Design review of the part built by this model. Coordinates are the model's own, in mm. Face numbers are marked on the shaded views. A direction names the side the tool comes from. Round coordinates to 2 decimals unless told otherwise and drop trailing zeros. Loops run counter-clockwise (first coordinate to the right, second up) from the corner with the lowest first, then second, coordinate; pieces in that order, holes last. Notation, with made-up numbers: M 23.25,36 L 52.25,36 A19 ccw 52.25,65 Z; hole C 62,58 d7. An arc over 180 degrees is marked long. Use a Markdown table: item, result.
from build123d import *

# Parameters (mm, degrees)
BOSS_EXTRU_1_DEPTH      = 10
ESQUISSE2_R             = 8.5
BOSS_EXTRU_2_DEPTH      = 15
BOSS_EXTRU_2_DEPTH_BACK = 25


with BuildPart() as part:
    # Esquisse1 → Boss.-Extru.1 (new body)
    with BuildSketch(Plane.XY):
        with BuildLine():
            Line((-38.999653337, 10.226454502), (-81.337427048, -4.313992939))
            ThreePointArc((-81.337427048, -4.313992939), (-86.130996021, -4.736088564), (-90.566704705, -2.870356351))
            Line((-90.566704705, -2.870356351), (-108.115218138, 10.226454502))
            ThreePointArc((-108.115218138, 10.226454502), (-118.115218138, 20.226454502), (-108.115218138, 30.226454502))
            Line((-108.115218138, 30.226454502), (61.31386316, 30.226454502))
            ThreePointArc((61.31386316, 30.226454502), (68.788631458, 33.322604906), (71.884781862, 40.797373204))
            Line((71.884781862, 40.797373204), (71.884781862, 45.226454502))
            ThreePointArc((71.884781862, 45.226454502), (81.607354933, 55.230528024), (91.884781862, 45.797373204))
            Line((91.884781862, 45.797373204), (91.884781862, 20.226454502))
            ThreePointArc((91.884781862, 20.226454502), (88.955849674, 13.15538669), (81.884781862, 10.226454502))
            Line((81.884781862, 10.226454502), (-38.999653337, 10.226454502))
        make_face()
    extrude(amount=BOSS_EXTRU_1_DEPTH)

    # Esquisse2 → Boss.-Extru.2 (add, two sides)
    with BuildSketch(Plane.XY.offset(10)) as boss_extru_2_sk:
        with Locations((-108.115218138, 20.226454502)):
            Circle(ESQUISSE2_R)
    extrude(amount=BOSS_EXTRU_2_DEPTH)
    extrude(boss_extru_2_sk.sketch, amount=-BOSS_EXTRU_2_DEPTH_BACK)


solid = part.part
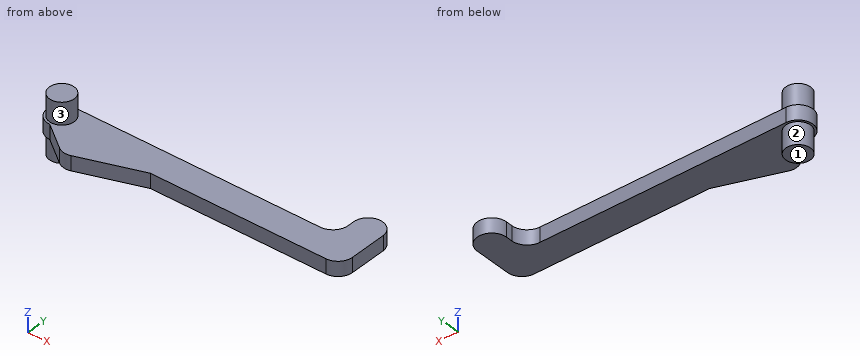
1. Insertion check: pin 1 (5 mm diameter, centred on x = 36, z = 3.5, fed in from -Y); pin 2 (2 mm diameter, centred on x = 71, y = 23, fed in from +Z); pin 3 (1.5 mm diameter, centred on y = 22.5, z = -1.5, fed in from -X). Each pin has a flat end and moves straight along its axis. Give the tip position at first contact, or say it passes through.
Check values:
| item | result |
|---|---|
| pin 1 | stops at y = 10.23 |
| pin 2 | stops at z = 10 |
| pin 3 | stops at x = -116.48 |
2. Take a section at D-D on x = -104.5. Give the boundary of the cut face in (y, z).
Check values:
| item | result |
|---|---|
| outline | M 7.53,0 L 12.53,0 L 12.53,-15 L 27.92,-15 L 27.92,0 L 30.23,0 L 30.23,10 L 27.92,10 L 27.92,25 L 12.53,25 L 12.53,10 L 7.53,10 Z |
3. Wall thickness on line 1 along Y through (x, z) = (48, 7.5); line 2 along Z through (x, y) = (75, 22); line 3 along X through (y, z) = (40.5, 2.5): over which ranges is each line inside the solid? List them lowest first. Write a range as from..to.
Check values:
| item | result |
|---|---|
| line 1 | y = 10.23..30.23 |
| line 2 | z = 0..10 |
| line 3 | x = 71.88..91.88 |
4. Take a section at C-C on y = 15. Give the boundary of the cut face in (x, z), and give its area (3 significant figures).
Check values:
| item | result |
|---|---|
| outline | M -116.64,0 L -114.82,0 L -114.82,-15 L -101.41,-15 L -101.41,0 L 90.41,0 L 90.41,10 L -101.41,10 L -101.41,25 L -114.82,25 L -114.82,10 L -116.64,10 Z |
| area | 2,470 mm² |
5. Machinability: for the marked faces 1, 2 and 3, which of the approach directions +Z, -Z, +X, -X, +Y, -Y give a long, thin tool a straight path to every point of the face, cutting with its end or side? Answer none if there is none.
Check values:
| item | result |
|---|---|
| face 1 | -Z, +X, -X, +Y, -Y |
| face 2 | -Z |
| face 3 | +Z |
6. Take a section at A-A on z = 5. Give the boundary of the cut face in (x, y).
Check values:
| item | result |
|---|---|
| outline | M -108.12,10.23 L -90.57,-2.87 A10 ccw -81.34,-4.31 L -39,10.23 L 81.88,10.23 A10 ccw 91.88,20.23 L 91.88,45.8 A10.01 ccw 71.88,45.23 L 71.88,40.8 A10.57 cw 61.31,30.23 L -108.12,30.23 A10 ccw Z |
7. Take a section at B-B on x = -31.5. Give the boundary of the cut face in (y, z).
Check values:
| item | result |
|---|---|
| outline | M 10.23,0 L 30.23,0 L 30.23,10 L 10.23,10 Z |
